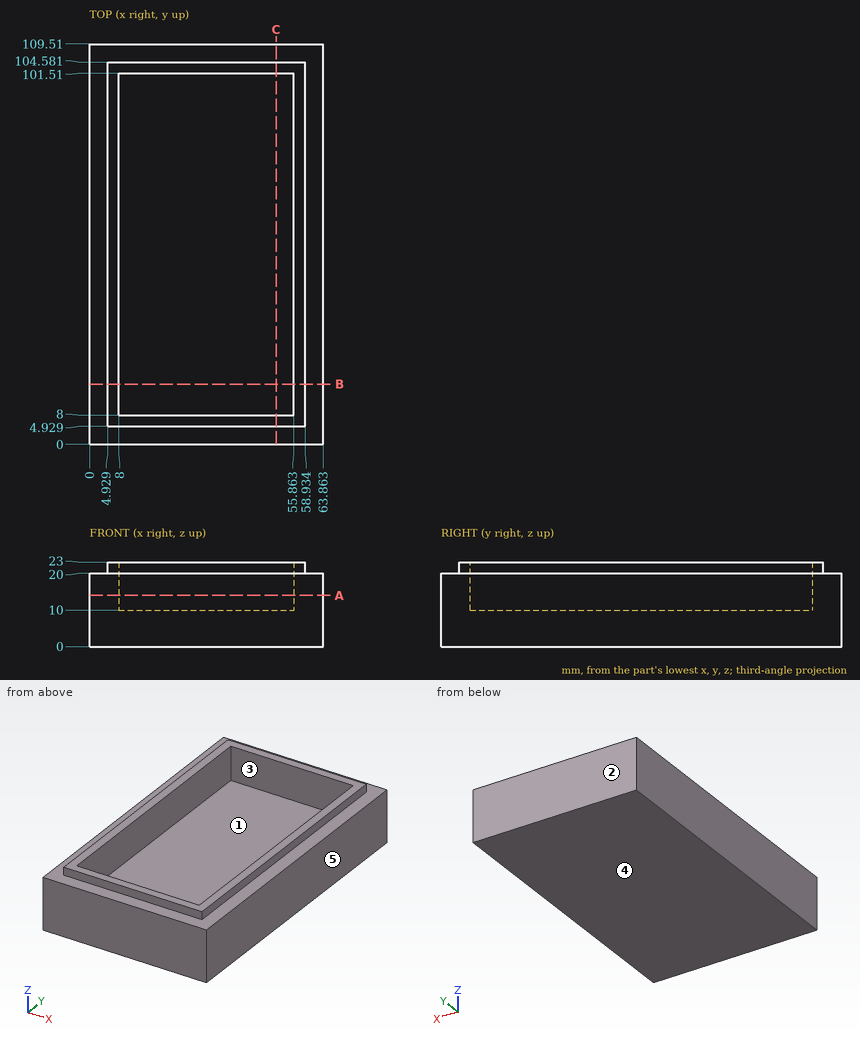
Here's the drawing with two shaded views (mm, measured from the low corner). I have some questions. A direction names the side the tool comes from. Give positions to 0.01 mm unless a question says otherwise; leave off trailing zeros. Order: outer loops, then holes, each group sorted by start corner. A loop starts at its lowest first (then second) coordinate and runs counter-clockwise, first axis right, second up. Notation, with made-up numbers: (-21.5, -21.5) - (15.5, -21.5) arc R29 ccw to (15.5, 4.5) - close; hole circle Ø5 at (-36, 80). An arc over 180 degrees is marked (long way). Write each question's results on one line, items separated by ' | '.
1) On a 3-axis mill with a long thin cutter (end or side, diameter ignored), from which of +Z, -Z, +X, -X, +Y, -Y can I reach the whole of each face in a straight line? I mean the marked faces 1 and 2. Say none if no direction works.
Final values:
face 1: +Z | face 2: +Z, -Z, +X, -X, +Y
2) Please list where these lines run through material, in increasing order: line 1 along X through (y, z) = (77.5, 12.5); line 2 along X through (y, z) = (64, 20.5); line 3 along Y through (x, z) = (22.5, 20.75). Write a range as [from, to].
Final values:
line 1: x = [0, 8], [55.86, 63.86] | line 2: x = [4.93, 8], [55.86, 58.93] | line 3: y = [4.93, 8], [101.51, 104.58]
3) Suppose I cut it at B-B, the plane y = 16.5. Write out the boundary of the cut face in (x, z), then the cut area to 3 significant figures.
Final values:
outline: (0, 0) - (63.86, 0) - (63.86, 20) - (58.93, 20) - (58.93, 23) - (55.86, 23) - (55.86, 10) - (8, 10) - (8, 23) - (4.93, 23) - (4.93, 20) - (0, 20) - close | area: 817 mm^2
4) Suppose I cut it at A-A, the plane z = 14. Write out the boundary of the cut face in (x, y).
Final values:
outline: (0, 0) - (63.86, 0) - (63.86, 109.51) - (0, 109.51) - close; hole (8, 8) - (55.86, 8) - (55.86, 101.51) - (8, 101.51) - close
5) I'm going to push flat-ended pins straight in: pin 1 Ø1.5 at (x, z) = (19, 22) entering from -Y; pin 2 Ø0.9 at (x, z) = (24.5, 21) entering from +Y; pin 3 Ø0.9 at (y, z) = (54.5, 21) entering from -X. Where does each tip first touch, or does it pass through?
Final values:
pin 1: stops at y = 4.93 | pin 2: stops at y = 104.58 | pin 3: stops at x = 4.93
6) Suppose I cut it at C-C, the plane x = 51. Write out the boundary of the cut face in (y, z).
Final values:
outline: (0, 0) - (109.51, 0) - (109.51, 20) - (104.58, 20) - (104.58, 23) - (101.51, 23) - (101.51, 10) - (8, 10) - (8, 23) - (4.93, 23) - (4.93, 20) - (0, 20) - close
7) If we mould it in two halves opening along X, with no side actions, what happens to the marked faces 3, 4 and 5? For each: pulls with the +X half, pulls with the -X half, needs draft (parallel to the pull), parting line crosses it, or undercut.
Final values:
face 3: undercut | face 4: needs draft | face 5: pulls with the +X half
